Part print with two shaded views. Sizes in mm from the minimum x, y, z corner. A direction names the side the tool comes from. Round coordinates to 2 decimals unless told otherwise and drop trailing zeros. Order: outer loops, then holes, each group sorted by start corner. A loop starts at its lowest first (then second) coordinate and runs counter-clockwise, first axis right, second up. Notation, with made-up numbers: (66, 19) -> (114, 19) arc R18 ccw to (114, 40) -> close; hole circle Ø4 at (36.5, 46.5). An arc over 180 degrees is marked (long way). Answer as a JSON object with one key per item and string values.
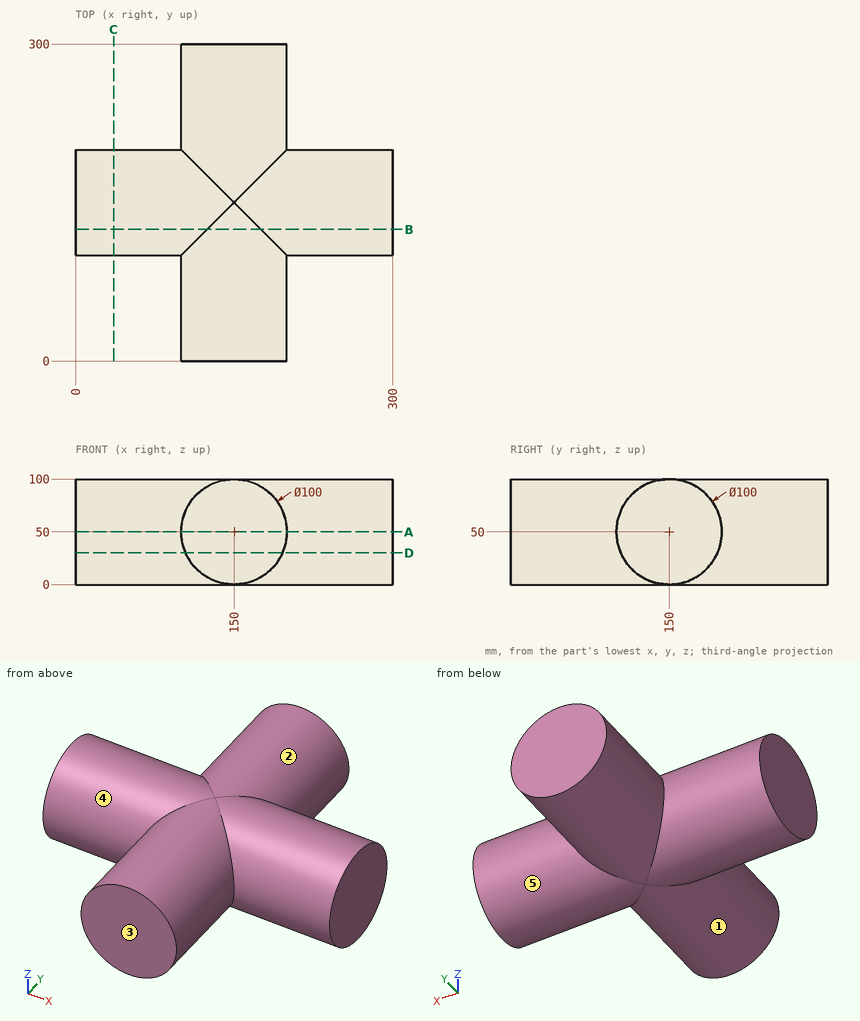
1) Which spindle directions (+Z, -Z, +X, -X, +Y, -Y) get a long thin tool onto all of the face, cutting with end or side? Do the marked faces 1, 2, 3, 4 and 5. Say none if no direction does.
Checked values:
{"face 1": "-Y", "face 2": "+Y", "face 3": "+Z, -Z, +X, -X, -Y", "face 4": "-X", "face 5": "+X"}
2) Cut at D-D, the plane z = 30. Give the cut face in (x, y).
Checked values:
{"outline": "(0, 104.17) -> (104.17, 104.17) -> (104.17, 0) -> (195.83, 0) -> (195.83, 104.17) -> (300, 104.17) -> (300, 195.83) -> (195.83, 195.83) -> (195.83, 300) -> (104.17, 300) -> (104.17, 195.83) -> (0, 195.83) -> close"}
3) Probe L1, parallel to Y at x = 82, z = 49; L2, parallel to X at y = 233, z = 48; L3, parallel to Y at x = 45, z = 19. List the from-to ranges inside material, lowest first. Write a range as from..to.
Checked values:
{"L1": "y = 100.01..199.99", "L2": "x = 100.04..199.96", "L3": "y = 110.77..189.23"}
4) Cut at B-B, the plane y = 124.5. Give the cut face in (x, z).
Checked values:
{"outline": "(0, 6.99) -> (124.5, 6.99) arc R50 ccw to (175.5, 6.99) -> (300, 6.99) -> (300, 93.01) -> (175.5, 93.01) arc R50 ccw to (124.5, 93.01) -> (0, 93.01) -> close"}
5) Cut at C-C, the plane x = 36. Give the cut face in (y, z).
Checked values:
{"outline": "circle Ø100 at (150, 50)"}
6) Flat gauge pins, fed straight in: pin 1 Ø5 at (x, z) = (31.5, 89) entering from -Y; pin 2 Ø2 at (x, z) = (86, 33.5) entering from +Y; pin 3 Ø2 at (x, y) = (123, 177) entering from -Z. Where does each tip first touch, or does it go through?
Checked values:
{"pin 1": "stops at y = 115.83", "pin 2": "stops at y = 197.54", "pin 3": "stops at z = 7.29"}
7) Cut at A-A, the plane z = 50. Give the cut face in (x, y).
Checked values:
{"outline": "(0, 100) -> (100, 100) -> (100, 0) -> (200, 0) -> (200, 100) -> (300, 100) -> (300, 200) -> (200, 200) -> (200, 300) -> (100, 300) -> (100, 200) -> (0, 200) -> close"}
